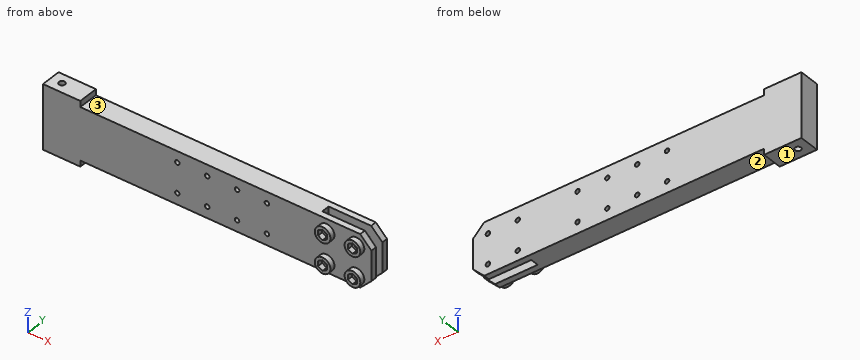
Autodesk Inventor part; units mm, degrees
ref_plane "Work Plane1" through (0, -2.75, 0) normal (0, -1, 0) x (1, 0, 0)
ref_plane "Work Plane2" through (-152.5, -8.5, -20) normal (0, 0, -1) x (-1, 0, 0)
ref_plane "Work Plane3" through (-195, -9.5, -21.5) normal (0, 0, -1) x (-1, 0, 0)
sketch "Sketch1" plane through (0, 0, 0) normal (0, 1, 0) x (-1, 0, 0)
  line L0 (0, 0) -> (220, 0)
  line L1 (220, 0) -> (220, -43)
  line L2 (220, -43) -> (0, -43)
  line L3 (0, -43) -> (0, 0)
  line L4 (10, -12.5) -> (30, -12.5)
  line L5 (30, -12.5) -> (30, -32.5)
  line L6 (30, -32.5) -> (10, -32.5)
  line L7 (10, -32.5) -> (10, -12.5)
  circle A0 centre (10, -12.5) radius 1.5
  circle A1 centre (30, -32.5) radius 1.5
  circle A2 centre (30, -12.5) radius 1.5
  circle A3 centre (10, -32.5) radius 1.5
  line L8 (220, 0) -> (195, 0)
  line L9 (195, 0) -> (195, -43)
  line L10 (195, -43) -> (220, -43)
  line L11 (220, -43) -> (220, 0)
  line L12 (195, -4) -> (0, -4)
  line L13 (0, -4) -> (0, -39)
  line L14 (0, -39) -> (195, -39)
  line L15 (195, -39) -> (195, -4)
  line L16 (36, -4) -> (36, -39)
  point P0 (195, 0)
  point P1 (0, -4)
  dimension "d0" = 220
  dimension "d1" = 43
  dimension "d2" = 20
  dimension "d3" = 20
  dimension "d4" = 12.5
  dimension "d5" = 10
  dimension "d6" = 3
  dimension "d7" = 3
  dimension "d8" = 3
  dimension "d9" = 3
  dimension "d18" = 4
  dimension "d19" = 4
  dimension "d23" = 36
  dimension "d66" = 25
extrude "Extrusion1" add sketch "Sketch1" along normal blind 4 contours L0 L1 L2 L9 | L12 L16 L14 L3 | L9 L14 L16 L12 | L4 A2 L5 A1 L6 A3 L7 A0
extrude "Extrusion2" add sketch "Sketch1" against normal blind 5.5 contours L0 L1 L2 L9 | L9 L14 L16 L12
ref_plane "Work Plane1" through (0, -2.75, 0) normal (0, -1, 0) x (1, 0, 0)
mirror "Mirror1" about plane through (0, -2.75, 0) normal (0, -1, 0) of "Extrusion1"
chamfer "Chamfer1" distance 7.5 angle 45 4 edges at (0, 2, -4) (0, -7.5, -4) (0, -7.5, -39) (0, 2, -39)
ref_plane "Work Plane2" through (-152.5, -8.5, -20) normal (0, 0, -1) x (-1, 0, 0)
sketch "Sketch5" plane through (-195, -9.5, -39) normal (0, -1, 0) x (1, 0, 0)
  circle A0 centre (165, 26.5) radius 1.5
  line L0 (165, 29.9641) -> (168, 28.2321)
  line L1 (168, 28.2321) -> (168, 24.7679)
  line L2 (168, 24.7679) -> (165, 23.0359)
  line L3 (165, 23.0359) -> (162, 24.7679)
  line L4 (162, 24.7679) -> (162, 28.2321)
  line L5 (162, 28.2321) -> (165, 29.9641)
  circle A1 centre (185, 26.5) radius 1.5
  line L6 (185, 29.9641) -> (188, 28.2321)
  line L7 (188, 28.2321) -> (188, 24.7679)
  line L8 (188, 24.7679) -> (185, 23.0359)
  line L9 (185, 23.0359) -> (182, 24.7679)
  line L10 (182, 24.7679) -> (182, 28.2321)
  line L11 (182, 28.2321) -> (185, 29.9641)
  circle A2 centre (185, 6.5) radius 1.5
  line L12 (185, 9.9641) -> (188, 8.2321)
  line L13 (188, 8.2321) -> (188, 4.7679)
  line L14 (188, 4.7679) -> (185, 3.0359)
  line L15 (185, 3.0359) -> (182, 4.7679)
  line L16 (182, 4.7679) -> (182, 8.2321)
  line L17 (182, 8.2321) -> (185, 9.9641)
  circle A3 centre (165, 6.5) radius 1.5
  line L18 (165, 9.9641) -> (168, 8.2321)
  line L19 (168, 8.2321) -> (168, 4.7679)
  line L20 (168, 4.7679) -> (165, 3.0359)
  line L21 (165, 3.0359) -> (162, 4.7679)
  line L22 (162, 4.7679) -> (162, 8.2321)
  line L23 (162, 8.2321) -> (165, 9.9641)
  circle A4 centre (165, 26.5) radius 5.25
  circle A5 centre (185, 26.5) radius 5.25
  circle A6 centre (185, 6.5) radius 5.25
  circle A7 centre (165, 6.5) radius 5.25
  point P0 (195, 39)
  dimension "d44" = 6
  dimension "d45" = 6
  dimension "d46" = 6
  dimension "d47" = 6
  dimension "d48" = 10.5
  dimension "d49" = 10.5
  dimension "d50" = 10.5
  dimension "d51" = 10.5
extrude "Extrusion5" add sketch "Sketch5" along normal blind 3.5 contours A4 | A5 | A6 | A7
sketch "Sketch6" plane through (-195, -9.5, -39) normal (0, -1, 0) x (1, 0, 0)
  circle A0 centre (65, 7.5) radius 1.5
  line L0 (187.5, 0) -> (0, 0)
  line L1 (0, 0) -> (0, -4)
  circle A1 centre (85, 7.5) radius 1.5
  circle A2 centre (105, 7.5) radius 1.5
  circle A3 centre (125, 7.5) radius 1.5
  point P0 (195, 39)
  point P1 (0, -5)
  dimension "d54" = 3
  dimension "d55" = 7.5
  dimension "d56" = 65
  dimension "d59" = 20
extrude "Extrusion6" cut sketch "Sketch6" against normal blind 33.25
ref_plane "Work Plane3" through (-195, -9.5, -21.5) normal (0, 0, -1) x (-1, 0, 0)
mirror "Mirror2" about plane through (-195, -9.5, -21.5) normal (0, 0, -1) of "Extrusion6"
sketch "Sketch7" plane through (-220, 4, 0) normal (0, 0, 1) x (1, 0, 0)
  point P0 (220, -4)
ref_plane "Work Plane4" through (-195, -9.5, -21.5) normal (0, 0, 1) x (1, 0, 0)
sketch "Sketch9" plane through (-220, 4, 0) normal (0, 0, 1) x (1, 0, 0)
  circle A0 centre (7.5, -6.75) radius 2
  line L0 (0, -13.5) -> (0, 0)
  line L1 (0, 0) -> (25, 0)
  point P0 (220, -4)
  dimension "d75" = 4
  dimension "d76" = 7.5
  dimension "d77" = 6.75
extrude "Extrusion8" cut sketch "Sketch9" against normal blind 73.25
properties part number "RobotBaseMotorExt"
Geometry: final body of the model. Coordinates: model frame, mm. Face numbers are marked on the shaded views. A direction names the side the tool comes from. Coordinates: 2 decimals unless noted, no trailing zeros. Order: outer loops, then holes, each group sorted by start corner. A loop starts at its lowest first (then second) coordinate and runs counter-clockwise, first axis right, second up. Notation, with made-up numbers: (-34.5, -7) - (-22.5, -7) arc R26 cw to (-22.5, 24) - close; hole circle Ø4 at (77, 0.5). An arc over 180 degrees is marked (long way). Return JSON: item names as keys, results as strings. Group by question number.
1. Cut plane C-C (x = -164.5). Output: boundary loops of the cut face in (y, z), plus the area to 4 significant figures.
2. Pin query (flat end, axial travel): pin 1 (5 mm diameter, centred on x = -30, z = -12.5, fed in from -Y); pin 2 (1.8 mm diameter, centred on x = -10, z = -32.5, fed in from +Y); pin 3 (2 mm diameter, centred on x = -158, y = -6.5, fed in from -Z); pin 4 (6.5 mm diameter, centred on x = -9, z = -12.5, fed in from -Y). Return the tip coordinate at first contact, or that it passes through.
3. Set-up query: the marked faces 1, 2 and 3. Return all of +Z, -Z, +X, -X, +Y, -Y with unobstructed straight access to the full face (end or side cutting, diameter ignored); none if empty.
4. Material intervals for line 1 along Z through (x, y) = (-130, -5); line 2 along Z through (x, y) = (-30, -7.15); line 3 along X through (y, z) = (-2.25, -11.5), sorted ascending. Write a range as [from, to].
5. Cut plane A-A (z = -24). Output: boundary loops of the cut face in (x, y).
6. Cut plane B-B (x = -212.5). Output: boundary loops of the cut face in (y, z), plus the area to 4 significant figures.
Resolved:
{
 "1": {"outline": "(-9.5, -39) - (4, -39) - (4, -4) - (-9.5, -4) - close", "area": "472.5 mm²"},
 "2": {"pin 1": "stops at y = -9.5", "pin 2": "passes through", "pin 3": "stops at z = -39", "pin 4": "stops at y = -13"},
 "3": {"face 1": "-Z, +X, -X, +Y, -Y", "face 2": "-Z, +X, +Y, -Y", "face 3": "+Z, +X, +Y, -Y"},
 "4": {"line 1": "z = [-39, -33], [-30, -13], [-10, -4]", "line 2": "z = [-39, -34], [-31, -14], [-11, -4]", "line 3": "x = [-220, -214.44], [-210.56, -131.5], [-128.5, -111.5], [-108.5, -91.5], [-88.5, -71.5], [-68.5, -36]"},
 "5": {"outline": "(-220, -9.5) - (0, -9.5) - (0, -5.5) - (-36, -5.5) - (-36, 0) - (0, 0) - (0, 4) - (-220, 4) - close; hole circle Ø4 at (-212.5, -2.75)"},
 "6": {"outline": "(-9.5, -43) - (-4.75, -43) - (-4.75, 0) - (-9.5, 0) - close; (-0.75, -43) - (4, -43) - (4, 0) - (-0.75, 0) - close", "area": "408.5 mm²"}
}
